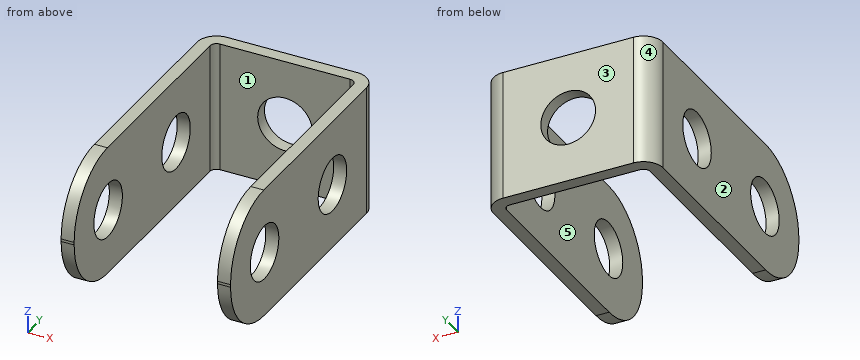
```python
from build123d import *

# Parameters (mm, degrees)
PAD_DEPTH       = 10
SKETCH002_R     = 2.1
POCKET_DEPTH    = 5
SKETCH001_R     = 2.1
POCKET001_DEPTH = 13.001
FILLET_R        = 4.9


with BuildPart() as part:
    # Sketch → Pad (new body)
    with BuildSketch(Plane.XY):
        with BuildLine():
            Line((0, -10), (0, 10))
            ThreePointArc((1.5, 11.5), (0.43934, 11.06066), (0, 10))
            Line((1.5, 11.5), (11.5, 11.5))
            ThreePointArc((13, 10), (12.56066, 11.06066), (11.5, 11.5))
            Line((13, 10), (13, -9.999991))
            Line((12, -9.999991), (13, -9.999991))
            Line((12, 10.000009), (12, -9.999991))
            ThreePointArc((12, 10.000009), (11.85355, 10.353556), (11.500001, 10.5))
            Line((1.5, 10.5), (11.500001, 10.5))
            ThreePointArc((1.5, 10.5), (1.146447, 10.353553), (1, 10))
            Line((1, -10), (1, 10))
            Line((0, -10), (1, -10))
        make_face()
    extrude(amount=PAD_DEPTH)

    # Sketch002 → Pocket (cut)
    with BuildSketch(Plane(origin=(0, 11.5, 0), x_dir=(-1, 0, 0), z_dir=(0, 1, 0))):
        with Locations((-6.5, 5)):
            Circle(SKETCH002_R)
    extrude(amount=-POCKET_DEPTH, mode=Mode.SUBTRACT)

    # Sketch001 → Pocket001 (cut, through all)
    with BuildSketch(Plane(origin=(0, 0, 0), x_dir=(0, -1, 0), z_dir=(-1, 0, 0))):
        with Locations((-5, 5)):
            Circle(SKETCH001_R)
        with Locations((5, 5)):
            Circle(SKETCH001_R)
    extrude(amount=-POCKET001_DEPTH, mode=Mode.SUBTRACT)

    # Fillet
    fillet_edges = [part.edges().sort_by_distance(p)[0] for p in [
        (0.5, -10, 10),
        (12.5, -9.999991, 10),
        (12.5, -9.999991, 0),
        (0.5, -10, 0),
    ]]
    fillet(fillet_edges, radius=FILLET_R)


solid = part.part
```
Read the model definition and answer for the solid it produces. Units are mm, in the model's axes. Face numbers are marked on the shaded views. A direction names the side the tool comes from. Coordinates: 2 decimals unless noted, no trailing zeros. Write each loop counter-clockwise with the first axis right and the second up, starting at its lowest first coordinate (ties: lowest second). Pieces come first, ordered by that corner, then holes. Notation, with made-up numbers: (-13.75, 64) - (27.25, 64) arc R14 cw to (27.25, 91) - close; hole circle Ø5 at (-26.5, 47.25). An arc over 180 degrees is marked (long way). Answer as a JSON object with one key per item and string values. Group by question number.
1. Which of the six approach directions +Z, -Z, +X, -X, +Y, -Y give full straight-line access (tool end or side, diameter ignored) to the marked faces 4 and 5?
2. A cutting plane is placed at A-A (y = 8.25). Determine the outline of the cut face in (x, z).
3. A cutting plane is placed at C-C (x = 6.5). Determine the outline of the cut face in (y, z), plus the area to 3 significant figures.
4. Consider L1, parallel to X at y = 1.25, z = 9; L2, parallel to Z at x = 0.4, y = -5; L3, parallel to Y at x = 4, z = 1.25. Determine where each line is inside the solid, lowest interval first. Write a range as [from, to].
5. A cutting plane is placed at B-B (y = 5). Determine the outline of the cut face in (x, z).
6. The mould has two halves that part along X. Classify the marked faces 1, 2 and 3: +X half, -X half, draft (parallel to the pull), parting line (faces both ways), or undercut.
7. A cutting plane is placed at D-D (z = 4.5). Give the number of separate pieces and of enclosed holes in the cut face, plus the area to 3 significant figures.
Worked out:
{
 "1": {"face 4": "+Z, -Z, -X, +Y", "face 5": "+Z, -Z, -Y"},
 "2": {"outline": "(0, 0) - (1, 0) - (1, 10) - (0, 10) - close; (12, 0) - (13, 0) - (13, 10) - (12, 10) - close"},
 "3": {"outline": "(10.5, 0) - (11.5, 0) - (11.5, 2.9) - (10.5, 2.9) - close; (10.5, 7.1) - (11.5, 7.1) - (11.5, 10) - (10.5, 10) - close", "area": "5.80 mm²"},
 "4": {"L1": "x = [0, 1], [12, 13]", "L2": "z = [0, 2.9], [7.1, 10]", "L3": "y = [10.5, 11.5]"},
 "5": {"outline": "(0, 0) - (1, 0) - (1, 2.9) - (0, 2.9) - close; (0, 7.1) - (1, 7.1) - (1, 10) - (0, 10) - close; (12, 0) - (13, 0) - (13, 2.9) - (12, 2.9) - close; (12, 7.1) - (13, 7.1) - (13, 10) - (12, 10) - close"},
 "6": {"face 1": "undercut", "face 2": "-X half", "face 3": "draft"},
 "7": {"separate pieces": "6", "enclosed holes": "0", "area": "32.7 mm²"}
}
